```python
from build123d import *

# Parameters (mm, degrees)
SKETCH1_R           = 2.5
SKETCH1_R_2         = 2.506016037
BOSS_EXTRUDE1_DEPTH = 2


with BuildPart() as part:
    # Sketch1 → Boss-Extrude1 (new body)
    with BuildSketch(Plane.XY):
        with BuildLine():
            Line((84.714565194, 13), (-84.714565194, 13))
            ThreePointArc((-84.714565194, 13), (-86.865323204, 12.765973581), (-88.915414375, 12.074847997))
            Line((-88.915414375, 12.074847997), (-103.401698361, 5.368984247))
            Line((-103.401698361, 5.368984247), (-103.860380263, 5.156655237))
            ThreePointArc((-103.860380263, 5.156655237), (-106.642942464, -0.456147767), (-101.759955673, -4.380768762))
            Line((-101.759955673, -4.380768762), (101.759955673, -4.380768762))
            ThreePointArc((101.759955673, -4.380768762), (106.642942464, -0.456147767), (103.860380263, 5.156655237))
            Line((103.860380263, 5.156655237), (88.915414375, 12.074847997))
            ThreePointArc((88.915414375, 12.074847997), (86.865323204, 12.765973581), (84.714565194, 13))
        make_face()
        with Locations((-100, 0)):
            Circle(SKETCH1_R, mode=Mode.SUBTRACT)
        with BuildLine():
            Line((-59.681677735, 1.761321711), (-56.14514104, -0.666672148))
            ThreePointArc((-56.14514104, -0.666672148), (-55.911681313, -1.339099386), (-56.484737706, -1.761317581))
            Line((-56.484737706, -1.761317581), (-91.130638371, -1.761317581))
            ThreePointArc((-91.130638371, -1.761317581), (-91.71541475, -1.295617942), (-91.392423967, -0.621439537))
            Line((-91.392423967, -0.621439537), (-86.478477199, 1.761321711))
            Line((-86.478477199, 1.761321711), (-59.681677735, 1.761321711))
        make_face(mode=Mode.SUBTRACT)
        with Locations((-50, 0)):
            Circle(SKETCH1_R, mode=Mode.SUBTRACT)
        with BuildLine():
            Line((-13.521523964, 1.761321711), (-8.607577196, -0.621439537))
            ThreePointArc((-8.607577196, -0.621439537), (-8.284586412, -1.295617942), (-8.869362791, -1.761317581))
            Line((-8.869362791, -1.761317581), (-43.515263456, -1.761317581))
            ThreePointArc((-43.515263456, -1.761317581), (-44.08831985, -1.339099386), (-43.854860123, -0.666672148))
            Line((-43.854860123, -0.666672148), (-40.318323427, 1.761321711))
            Line((-40.318323427, 1.761321711), (-13.521523964, 1.761321711))
        make_face(mode=Mode.SUBTRACT)
        Circle(SKETCH1_R_2, mode=Mode.SUBTRACT)
        with BuildLine():
            Line((40.318323427, 1.761321711), (43.854860123, -0.666672148))
            ThreePointArc((43.854860123, -0.666672148), (44.08831985, -1.339099386), (43.515263456, -1.761317581))
            Line((43.515263456, -1.761317581), (8.869362791, -1.761317581))
            ThreePointArc((8.869362791, -1.761317581), (8.284586412, -1.295617942), (8.607577196, -0.621439537))
            Line((8.607577196, -0.621439537), (13.521523964, 1.761321711))
            Line((13.521523964, 1.761321711), (40.318323427, 1.761321711))
        make_face(mode=Mode.SUBTRACT)
        with Locations((50.000000581, 2.065e-06)):
            Circle(SKETCH1_R, mode=Mode.SUBTRACT)
        with BuildLine():
            Line((86.478477199, 1.761321711), (91.392423967, -0.621439537))
            ThreePointArc((91.392423967, -0.621439537), (91.71541475, -1.295617942), (91.130638371, -1.761317581))
            Line((91.130638371, -1.761317581), (56.484737706, -1.761317581))
            ThreePointArc((56.484737706, -1.761317581), (55.911681313, -1.339099386), (56.14514104, -0.666672148))
            Line((56.14514104, -0.666672148), (59.681677735, 1.761321711))
            Line((59.681677735, 1.761321711), (86.478477199, 1.761321711))
        make_face(mode=Mode.SUBTRACT)
        with Locations((100, 0)):
            Circle(SKETCH1_R, mode=Mode.SUBTRACT)
        with BuildLine():
            ThreePointArc((-86.478477199, 9.004514969), (-84.681411012, 9.523161606), (-82.81919634, 9.698083666))
            Line((-82.81919634, 9.698083666), (82.81919634, 9.698083666))
            ThreePointArc((82.81919634, 9.698083666), (84.681411012, 9.523161606), (86.478477199, 9.004514969))
            Line((86.478477199, 9.004514969), (88.830674001, 8.079633191))
            ThreePointArc((88.830674001, 8.079633191), (89.200621826, 7.409514432), (88.611117149, 6.921247313))
            Line((88.611117149, 6.921247313), (84.714565194, 6.921247313))
            Line((84.714565194, 6.921247313), (-84.714565194, 6.921247313))
            Line((-84.714565194, 6.921247313), (-88.611117149, 6.921247313))
            ThreePointArc((-88.611117149, 6.921247313), (-89.200621826, 7.409514432), (-88.830674001, 8.079633191))
            Line((-88.830674001, 8.079633191), (-86.478477199, 9.004514969))
        make_face(mode=Mode.SUBTRACT)
    extrude(amount=BOSS_EXTRUDE1_DEPTH)


solid = part.part
```
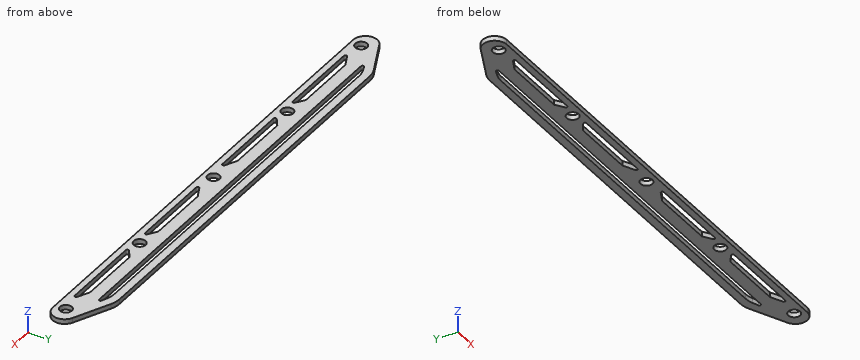
Source: CAD feature listing. Evaluate the final solid. Frame: model axes, mm. Coordinates: 2 decimals unless noted, no trailing zeros. Write each loop counter-clockwise with the first axis right and the second up, starting at its lowest first coordinate (ties: lowest second). Pieces come first, ordered by that corner, then holes. Notation, with made-up numbers: (-31, 5.25) -> (-2, 5.25) arc R15 cw to (-2, 30.25) -> close; hole circle Ø2 at (52, -37.75). An arc over 180 degrees is marked (long way). Return JSON: item names as keys, results as strings. Group by question number.
1) Ray query, line 1 along Y through (x, z) = (-50, 0.5); line 2 along Y through (x, z) = (-71.5, 0.6); line 3 along Y through (x, z) = (100, 1). Return the intervals inside material, ascending.
2) Section query C-C, the plane z = 1.6. State how many separate pieces and enclosed holes the cut face has, plus the area to 3 significant figures.
3) Section query A-A, the plane x = 0. Return loops of the section in (y, z).
4) Section query D-D, the plane x = 100. Return loops of the section in (y, z).
5) Section query B-B, the plane x = 50. Return loops of the section in (y, z), plus the area to 3 significant figures.
From the geometry:
{
 "1": {"line 1": "-4.38 to -2.5, 2.5 to 6.92, 9.7 to 13", "line 2": "-4.38 to -1.76, 1.76 to 6.92, 9.7 to 13", "line 3": "-4.38 to -2.5, 2.5 to 6.94"},
 "2": {"separate pieces": "1", "enclosed holes": "10", "area": "2,470 mm²"},
 "3": {"outline": "(-4.38, 0) -> (-2.51, 0) -> (-2.51, 2) -> (-4.38, 2) -> close; (2.51, 0) -> (6.92, 0) -> (6.92, 2) -> (2.51, 2) -> close; (9.7, 0) -> (13, 0) -> (13, 2) -> (9.7, 2) -> close"},
 "4": {"outline": "(-4.38, 0) -> (-2.5, 0) -> (-2.5, 2) -> (-4.38, 2) -> close; (2.5, 0) -> (6.94, 0) -> (6.94, 2) -> (2.5, 2) -> close"},
 "5": {"outline": "(-4.38, 0) -> (-2.5, 0) -> (-2.5, 2) -> (-4.38, 2) -> close; (2.5, 0) -> (6.92, 0) -> (6.92, 2) -> (2.5, 2) -> close; (9.7, 0) -> (13, 0) -> (13, 2) -> (9.7, 2) -> close", "area": "19.2 mm²"}
}
